from build123d import *

# Parameters (mm, degrees)
BOSS_EXTRUDE1_DEPTH = 25.4


with BuildPart() as part:
    # Sketch1 → Boss-Extrude1 (new body)
    with BuildSketch(Plane.XY):
        Polygon((12.7, 25.4), (0, 25.4), (0, 0), (63.5, 0), (63.5, 12.7), (44.45, 12.7), (44.45, 25.4), (25.4, 25.4), (25.4, 15.875), (12.7, 15.875), align=None)
        with BuildLine():
            Line((36.83, 19.05), (36.83, 6.35))
            ThreePointArc((36.83, 6.35), (34.925, 4.445), (33.02, 6.35))
            Line((33.02, 6.35), (33.02, 19.05))
            ThreePointArc((33.02, 19.05), (34.925, 20.955), (36.83, 19.05))
        make_face(mode=Mode.SUBTRACT)
    extrude(amount=-BOSS_EXTRUDE1_DEPTH)


solid = part.part
Model file for the job. Use its own axes, mm. A direction names the side the tool comes from. Give positions to 0.01 mm unless a question says otherwise; leave off trailing zeros. Loops run counter-clockwise (first coordinate to the right, second up) from the corner with the lowest first, then second, coordinate; pieces in that order, holes last.
1) Flat gauge pins, fed straight in: pin 1 Ø7.5 at (y, z) = (21.5, -14) entering from +X; pin 2 Ø4 at (x, z) = (21.5, -17.5) entering from +Y (3 decimals); pin 3 Ø9.5 at (x, z) = (56, -9.5) entering from +Y. Where does each tip first touch, or does it go through?
2) Saw through at D-D (x = 15.5). Write the cut outline in (y, z) (3 decimals).
3) Pull direction X, two halves, no side cores. Call faces 6 (the flat face through (63.5, 6, -13)), 7 (the flat face through (35, 25.4, -13)), 8 (the flat face through (25.4, 21, -13)): +X half, -X half, draft (parallel to the pull), parting line (faces both ways), or undercut.
4) Saw through at B-B (z = -12.75). Write the cut outline in (x, y) (3 decimals).
5) Wall check: line 1 (X direction, y = 19, z = -18.5); line 2 (X direction, y = 13.5, z = -15.75); line 3 (Y direction, x = 35, z = -23.5). Give the ranges that are in metal, low to high.
6) Saw through at A-A (y = 9.75). Write the cut outline in (x, z).
7) Saw through at C-C (x = 35). Write the cut outline in (y, z).
8) Tool access for faces 1 (the flat face through (24, 10, -25.4)), 2 (the flat face through (0, 13, -13)), 3 (the flat face through (19, 15.875, -13)), 4 (the flat face through (36.83, 13, -13)), 5 (the flat face through (44.45, 19, -13)): list every direction of +Z, -Z, +X, -X, +Y, -Y with a clear straight run to the whole face (end or side of a thin tool).
Answer block:
1. pin 1: stops at x = 44.45
1. pin 2: stops at y = 15.875
1. pin 3: stops at y = 12.7
2. outline: (0, -25.4) - (15.875, -25.4) - (15.875, 0) - (0, 0) - close
3. face 6: +X half
3. face 7: draft
3. face 8: undercut
4. outline: (0, 0) - (63.5, 0) - (63.5, 12.7) - (44.45, 12.7) - (44.45, 25.4) - (25.4, 25.4) - (25.4, 15.875) - (12.7, 15.875) - (12.7, 25.4) - (0, 25.4) - close; hole (33.02, 6.35) arc R1.905 ccw to (36.83, 6.35) - (36.83, 19.05) arc R1.905 ccw to (33.02, 19.05) - close
5. line 1: x = 0 to 12.7, 25.4 to 33.02, 36.83 to 44.45
5. line 2: x = 0 to 33.02, 36.83 to 44.45
5. line 3: y = 0 to 4.45, 20.95 to 25.4
6. outline: (0, -25.4) - (33.02, -25.4) - (33.02, 0) - (0, 0) - close; (36.83, -25.4) - (63.5, -25.4) - (63.5, 0) - (36.83, 0) - close
7. outline: (0, -25.4) - (4.45, -25.4) - (4.45, 0) - (0, 0) - close; (20.95, -25.4) - (25.4, -25.4) - (25.4, 0) - (20.95, 0) - close
8. face 1: -Z, +X, -X, +Y, -Y
8. face 2: +Z, -Z, -X, +Y, -Y
8. face 3: +Z, -Z, +Y
8. face 4: +Z, -Z
8. face 5: +Z, -Z, +X, +Y
